Autodesk Inventor part; units mm, degrees
ref_plane "YZ Plane" through (0, 0, 0) normal (1, 0, 0) x (0, 1, 0)
ref_plane "XZ Plane" through (0, 0, 0) normal (0, 1, 0) x (-1, 0, 0)
ref_plane "XY Plane" through (0, 0, 0) normal (0, 0, 1) x (1, 0, 0)
sketch "Skizze1" plane through (0, 0, 0) normal (0, 0, 1) x (1, 0, 0)
  line L0 (-21, 0) -> (21, 0)
  line L1 (0, -8.4) -> (0, 8.4)
  line L2 (15, -6) -> (-15, -6)
  line L3 (-15, -6) -> (-15, 6)
  line L4 (-15, 6) -> (15, 6)
  line L5 (15, 6) -> (15, -6)
  line L6 (15, -6) -> (-15, 6) construction
  line L7 (-15, -6) -> (15, 6) construction
  point P0 (0, 0)
  dimension "d0" = 12
  dimension "d1" = 30
extrude "Extrusion1" add sketch "Skizze1" along normal blind 4
sketch "Skizze2" plane through (0, 0, 0) normal (0, 0, -1) x (-1, 0, 0)
  line L0 (15, -6) -> (-15, -6)
  line L1 (15, 6) -> (15, -6)
  line L2 (-15, 6) -> (15, 6)
  line L3 (21, 0) -> (-21, 0)
  line L4 (0, -8.4) -> (0, 8.4)
  point P0 (0, 0)
  point P1 (-1, 0)
  point P2 (11, 0)
  point P3 (15, 0)
  dimension "d5" = 4
  dimension "d6" = 16
hole "Bohrung1" at (1, 0, 0) at (-11, 0, 0) direction (0, 0, 1) diameter 4.5 end through all
sketch "Skizze3" plane through (0, 0, 4) normal (0, 0, 1) x (1, 0, 0)
  circle A0 centre (-11, 0) radius 2.25
  circle A1 centre (1, 0) radius 2.25
  line L0 (-15, -6) -> (15, -6)
  line L1 (15, -6) -> (15, 6)
  line L2 (15, 6) -> (-15, 6)
  line L3 (-15, 6) -> (-15, -6)
  line L4 (-21, 0) -> (21, 0)
  line L5 (0, -8.4) -> (0, 8.4)
  point P0 (0, 0)
  point P1 (12, 0)
  dimension "d14" = 3
hole "Bohrung2" at (12, 0, 4) direction (0, 0, -1) diameter 3.242 end through all
sketch "Skizze4" plane through (0, 0, 4) normal (0, 0, 1) x (1, 0, 0)
  circle A0 centre (12, 0) radius 1.621
  circle A1 centre (-11, 0) radius 2.25
  circle A2 centre (1, 0) radius 2.25
  line L0 (-15, -6) -> (15, -6)
  line L1 (15, -6) -> (15, 6)
  line L2 (15, 6) -> (-15, 6)
  line L3 (-15, 6) -> (-15, -6)
  line L4 (-11, 2.25) -> (1, 2.25)
  line L5 (1, 2.25) -> (1, -2.25)
  line L6 (1, -2.25) -> (-11, -2.25)
  line L7 (-11, -2.25) -> (-11, 2.25)
  circle A3 centre (1, 0) radius 2.25
  point P0 (0, 0)
extrude "Extrusion2" cut sketch "Skizze4" against normal through all contours A1 L4 A2 L6
properties part number "24_0497_0021"
The model under review builds one solid part; all positions refer to its coordinate system, in mm. A direction names the side the tool comes from. Give positions to 0.01 mm unless a question says otherwise; leave off trailing zeros. Write each loop counter-clockwise with the first axis right and the second up, starting at its lowest first coordinate (ties: lowest second). Pieces come first, ordered by that corner, then holes. Notation, with made-up numbers: (3.5, 71.25) - (25.5, 71.25) arc R30 ccw to (25.5, 106.25) - close; hole circle Ø2 at (-37, -37). An arc over 180 degrees is marked (long way). Answer in a Markdown table with one row per item. Add a question column.
1. Draft analysis for pull direction X (two halves, no side actions). For faces 1 (the flat face through (-15, 0, 2)), 2 (the flat face through (15, 0, 2)), 3 (the flat face through (0, 6, 2)), 4 (the cylindrical face through (10.393, 0.211, 1.972)), state which applies: +X half, -X half, draft (parallel to the pull), parting line (faces both ways), or undercut.
2. We need section B-B on x = 12. Write out the cut boundary in (y, z), then the cut area to 3 significant figures.
3. We need section D-D on y = 1.25. Write out the cut boundary in (x, z).
4. Wall thickness on line 1 along X through (y, z) = (0, 1.6); line 2 along Y through (x, z) = (12, 1.8); line 3 along X through (y, z) = (1, 2.3): over which ranges is each line inside the solid? List them lowest first. Write a range as [from, to].
5. We need section A-A on y = 0. Write out the cut boundary in (x, z).
6. Tool access review of faces 5 (the flat face through (-5, -2.25, 2)), 6 (the flat face through (0, 3, 0)): name each direction out of +Z, -Z, +X, -X, +Y, -Y from which nothing blocks a thin tool from reaching the whole face with its end or side.
7. We need section C-C on z = 1.9. Write out the cut boundary in (x, y).
Ans:
| question | item | result |
|---|---|---|
| 1 | face 1 | -X half |
| 1 | face 2 | +X half |
| 1 | face 3 | draft |
| 1 | face 4 | undercut |
| 2 | outline | (-6, 0) - (-1.62, 0) - (-1.62, 4) - (-6, 4) - close; (1.62, 0) - (6, 0) - (6, 4) - (1.62, 4) - close |
| 2 | area | 35.0 mm^2 |
| 3 | outline | (-15, 0) - (-12.87, 0) - (-12.87, 4) - (-15, 4) - close; (2.87, 0) - (10.97, 0) - (10.97, 4) - (2.87, 4) - close; (13.03, 0) - (15, 0) - (15, 4) - (13.03, 4) - close |
| 4 | line 1 | x = [-15, -13.25], [3.25, 10.38], [13.62, 15] |
| 4 | line 2 | y = [-6, -1.62], [1.62, 6] |
| 4 | line 3 | x = [-15, -13.02], [3.02, 10.72], [13.28, 15] |
| 5 | outline | (-15, 0) - (-13.25, 0) - (-13.25, 4) - (-15, 4) - close; (3.25, 0) - (10.38, 0) - (10.38, 4) - (3.25, 4) - close; (13.62, 0) - (15, 0) - (15, 4) - (13.62, 4) - close |
| 6 | face 5 | +Z, -Z |
| 6 | face 6 | -Z, +X, -X, +Y, -Y |
| 7 | outline | (-15, -6) - (15, -6) - (15, 6) - (-15, 6) - close; hole (-11, -2.25) - (1, -2.25) arc R2.25 ccw to (1, 2.25) - (-11, 2.25) arc R2.25 ccw to start; hole circle Ø3.24 at (12, 0) |
